from build123d import *

# Parameters (mm, degrees)
CYLINDER002_R             = 3
CYLINDER002_DEPTH         = 10
BOX040_W                  = 56
BOX040_H                  = 10
BOX040_DEPTH              = 122
BOX021_W                  = 47.2
BOX021_H                  = 35
BOX021_DEPTH              = 8
BOX023_W                  = 4.5
BOX023_H                  = 2
BOX023_DEPTH              = 8
BOX022_W                  = 2
BOX022_H                  = 4.5
BOX022_DEPTH              = 8
BOX020_W                  = 17
BOX020_H                  = 5
BOX020_DEPTH              = 12
BOX018_W                  = 48.5
BOX018_H                  = 4.6
BOX018_DEPTH              = 25.5
FUSION005_PLACEMENT_ANGLE = 90
BOX029_W                  = 10
BOX029_H                  = 5
BOX029_DEPTH              = 10
BOX027_W                  = 29.6
BOX027_H                  = 2
BOX027_DEPTH              = 99.5
BOX028_W                  = 10
BOX028_H                  = 5
BOX028_DEPTH              = 10
BOX035_W                  = 10
BOX035_H                  = 77
BOX035_DEPTH              = 10
BOX034_W                  = 10
BOX034_H                  = 74
BOX034_DEPTH              = 10
CUT016_PLACEMENT_ANGLE    = 90
BOX037_W                  = 10
BOX037_H                  = 77
BOX037_DEPTH              = 10
BOX036_W                  = 10
BOX036_H                  = 74
BOX036_DEPTH              = 10
CUT017_PLACEMENT_ANGLE    = 90
BOX039_W                  = 10
BOX039_H                  = 77
BOX039_DEPTH              = 10
BOX038_W                  = 10
BOX038_H                  = 74
BOX038_DEPTH              = 10
CUT018_PLACEMENT_ANGLE    = 180
BOX033_W                  = 10
BOX033_H                  = 77
BOX033_DEPTH              = 10
BOX017_W                  = 10
BOX017_H                  = 74
BOX017_DEPTH              = 10
BOX032_W                  = 39
BOX032_H                  = 10
BOX032_DEPTH              = 10
BOX024_W                  = 50
BOX024_H                  = 39
BOX024_DEPTH              = 8
BOX026_W                  = 72
BOX026_H                  = 18
BOX026_DEPTH              = 1.7
BOX025_W                  = 3
BOX025_H                  = 10
BOX025_DEPTH              = 5.8
ARRAY005_X_COUNT          = 2
ARRAY005_X_PITCH          = 67
CYLINDER001_R             = 1.2
CYLINDER001_DEPTH         = 4
CYLINDER_R                = 2.6
CYLINDER_DEPTH            = 4
ARRAY006_X_COUNT          = 2
ARRAY006_X_PITCH          = 25
ARRAY006_Z_COUNT          = 2
ARRAY006_Z_PITCH          = 95
BOX016_W                  = 114
BOX016_H                  = 50
BOX016_DEPTH              = 144
BOX015_W                  = 120
BOX015_H                  = 42
BOX015_DEPTH              = 150
FILLET001_R               = 7
CHAMFER_SIZE              = 5
FILLET002_R               = 1.5


with BuildPart() as cilindro002:
    # Cylinder002 → Cylinder002 (new body)
    with BuildSketch(Plane(origin=(101.22, 63.68, 142.21), x_dir=(1, 0, 0), z_dir=(0, 0, 1))):
        Circle(CYLINDER002_R)
    extrude(amount=CYLINDER002_DEPTH)


with BuildPart() as cubo021:
    # Box040 → Box040 (new body)
    with BuildSketch(Plane(origin=(11, 81, 19), x_dir=(1, 0, 0), z_dir=(0, 0, 1))):
        with Locations((28, 5)):
            Rectangle(BOX040_W, BOX040_H)
    extrude(amount=BOX040_DEPTH)


with BuildPart() as protoboard:
    # Box021 → Box021 (new body)
    with BuildSketch(Plane.XY):
        with Locations((23.6, 17.5)):
            Rectangle(BOX021_W, BOX021_H)
    extrude(amount=BOX021_DEPTH)


with BuildPart() as obj1:
    # Box023 → Box023 (new body)
    with BuildSketch(Plane(origin=(21.25, 35, 0), x_dir=(1, 0, 0), z_dir=(0, 0, 1))):
        with Locations((2.25, 1)):
            Rectangle(BOX023_W, BOX023_H)
    extrude(amount=BOX023_DEPTH)


with BuildPart() as obj2:
    # Box022 → Box022 (new body)
    with BuildSketch(Plane(origin=(47, 15.25, 0), x_dir=(1, 0, 0), z_dir=(0, 0, 1))):
        with Locations((1, 2.25)):
            Rectangle(BOX022_W, BOX022_H)
    extrude(amount=BOX022_DEPTH)


with BuildPart() as cubo010:
    # Box020 → Box020 (new body)
    with BuildSketch(Plane(origin=(-7, 5, 6.75), x_dir=(1, 0, 0), z_dir=(0, 0, 1))):
        with Locations((8.5, 2.5)):
            Rectangle(BOX020_W, BOX020_H)
    extrude(amount=BOX020_DEPTH)


with BuildPart() as obj3:
    # Box018 → Box018 (new body)
    with BuildSketch(Plane(origin=(0, 0.4, 0), x_dir=(1, 0, 0), z_dir=(0, 0, 1))):
        with Locations((24.25, 2.3)):
            Rectangle(BOX018_W, BOX018_H)
    extrude(amount=BOX018_DEPTH)

    # Fusion005: union Cubo010
    add(cubo010.part)


with BuildPart() as obj3_1:
    # Fusion005 placement: moved
    add(obj3.part.moved(Location((-0.75, 30.25, 7.6))).rotate(Axis((-0.75, 30.25, 7.6), (1, 0, 0)), FUSION005_PLACEMENT_ANGLE))

    # Fusion006: union protoboard, obj1, obj2
    add(protoboard.part)
    add(obj1.part)
    add(obj2.part)


with BuildPart() as obj3_2:
    # Fusion006 placement: moved
    add(obj3_1.part.moved(Location((4, 45, 3))))


with BuildPart() as on_off:
    # Box029 → Box029 (new body)
    with BuildSketch(Plane(origin=(26, -6, 81.5), x_dir=(1, 0, 0), z_dir=(0, 0, 1))):
        with Locations((5, 2.5)):
            Rectangle(BOX029_W, BOX029_H)
    extrude(amount=BOX029_DEPTH)


with BuildPart() as obj4:
    # Box027 → Box027 (new body)
    with BuildSketch(Plane.XY):
        with Locations((14.8, 1)):
            Rectangle(BOX027_W, BOX027_H)
    extrude(amount=BOX027_DEPTH)


with BuildPart() as fusion011:
    # Box028 → Box028 (new body)
    with BuildSketch(Plane(origin=(26, 0.6, 5.5), x_dir=(1, 0, 0), z_dir=(0, 0, 1))):
        with Locations((5, 2.5)):
            Rectangle(BOX028_W, BOX028_H)
    extrude(amount=BOX028_DEPTH)

    # Fusion008: union on_off, obj4
    add(on_off.part)
    add(obj4.part)


with BuildPart() as fusion011_1:
    # Fusion008 placement: moved
    add(fusion011.part.moved(Location((85.8, 76, 4.23))))

    # Fusion011: union obj3
    add(obj3_2.part)


with BuildPart() as cubo016:
    # Box035 → Box035 (new body)
    with BuildSketch(Plane(origin=(0, 10, 140), x_dir=(1, 0, 0), z_dir=(0, 0, 1))):
        with Locations((5, 38.5)):
            Rectangle(BOX035_W, BOX035_H)
    extrude(amount=BOX035_DEPTH)


with BuildPart() as cut016:
    # Box034 → Box034 (new body)
    with BuildSketch(Plane(origin=(-3, 10, 143), x_dir=(1, 0, 0), z_dir=(0, 0, 1))):
        with Locations((5, 37)):
            Rectangle(BOX034_W, BOX034_H)
    extrude(amount=BOX034_DEPTH)

    # Cut016: cut Cubo016
    add(cubo016.part, mode=Mode.SUBTRACT)


with BuildPart() as cut016_1:
    # Cut016 placement: moved
    add(cut016.part.moved(Location((-30, 0, 150))).rotate(Axis((-30, 0, 150), (0, 1, 0)), CUT016_PLACEMENT_ANGLE))


with BuildPart() as cubo018:
    # Box037 → Box037 (new body)
    with BuildSketch(Plane(origin=(0, 10, 140), x_dir=(1, 0, 0), z_dir=(0, 0, 1))):
        with Locations((5, 38.5)):
            Rectangle(BOX037_W, BOX037_H)
    extrude(amount=BOX037_DEPTH)


with BuildPart() as cut017:
    # Box036 → Box036 (new body)
    with BuildSketch(Plane(origin=(-3, 10, 143), x_dir=(1, 0, 0), z_dir=(0, 0, 1))):
        with Locations((5, 37)):
            Rectangle(BOX036_W, BOX036_H)
    extrude(amount=BOX036_DEPTH)

    # Cut017: cut Cubo018
    add(cubo018.part, mode=Mode.SUBTRACT)


with BuildPart() as cut017_1:
    # Cut017 placement: moved
    add(cut017.part.moved(Location((150, 0, 0))).rotate(Axis((150, 0, 0), (0, -1, 0)), CUT017_PLACEMENT_ANGLE))


with BuildPart() as cubo020:
    # Box039 → Box039 (new body)
    with BuildSketch(Plane(origin=(0, 10, 140), x_dir=(1, 0, 0), z_dir=(0, 0, 1))):
        with Locations((5, 38.5)):
            Rectangle(BOX039_W, BOX039_H)
    extrude(amount=BOX039_DEPTH)


with BuildPart() as cut018:
    # Box038 → Box038 (new body)
    with BuildSketch(Plane(origin=(-3, 10, 143), x_dir=(1, 0, 0), z_dir=(0, 0, 1))):
        with Locations((5, 37)):
            Rectangle(BOX038_W, BOX038_H)
    extrude(amount=BOX038_DEPTH)

    # Cut018: cut Cubo020
    add(cubo020.part, mode=Mode.SUBTRACT)


with BuildPart() as cut018_1:
    # Cut018 placement: moved
    add(cut018.part.moved(Location((120, 0, 150))).rotate(Axis((120, 0, 150), (0, 1, 0)), CUT018_PLACEMENT_ANGLE))


with BuildPart() as cubo014:
    # Box033 → Box033 (new body)
    with BuildSketch(Plane(origin=(0, 10, 140), x_dir=(1, 0, 0), z_dir=(0, 0, 1))):
        with Locations((5, 38.5)):
            Rectangle(BOX033_W, BOX033_H)
    extrude(amount=BOX033_DEPTH)


with BuildPart() as obj5:
    # Box017 → Box017 (new body)
    with BuildSketch(Plane(origin=(-3, 10, 143), x_dir=(1, 0, 0), z_dir=(0, 0, 1))):
        with Locations((5, 37)):
            Rectangle(BOX017_W, BOX017_H)
    extrude(amount=BOX017_DEPTH)

    # Cut015: cut Cubo014
    add(cubo014.part, mode=Mode.SUBTRACT)

    # Fusion009: union Cut016, Cut017, Cut018
    add(cut016_1.part)
    add(cut017_1.part)
    add(cut018_1.part)


with BuildPart() as cubo013:
    # Box032 → Box032 (new body)
    with BuildSketch(Plane(origin=(9, 43, 3), x_dir=(1, 0, 0), z_dir=(0, 0, 1))):
        with Locations((19.5, 5)):
            Rectangle(BOX032_W, BOX032_H)
    extrude(amount=BOX032_DEPTH)


with BuildPart() as baseproto:
    # Box024 → Box024 (new body)
    with BuildSketch(Plane(origin=(3, 43, 3), x_dir=(1, 0, 0), z_dir=(0, 0, 1))):
        with Locations((25, 19.5)):
            Rectangle(BOX024_W, BOX024_H)
    extrude(amount=BOX024_DEPTH)

    # Cut014: cut Cubo013
    add(cubo013.part, mode=Mode.SUBTRACT)


with BuildPart() as leds:
    # Box026 → Box026 (new body)
    with BuildSketch(Plane(origin=(-1, 0, 2), x_dir=(1, 0, 0), z_dir=(0, 0, 1))):
        with Locations((36, 9)):
            Rectangle(BOX026_W, BOX026_H)
    extrude(amount=BOX026_DEPTH)


with BuildPart() as soporte_placa_leds:
    # Box025 → Box025 (new body)
    with BuildSketch(Plane(origin=(0, 8, 0), x_dir=(1, 0, 0), z_dir=(0, 0, 1))):
        with Locations((1.5, 5)):
            Rectangle(BOX025_W, BOX025_H)
    extrude(amount=BOX025_DEPTH)

    # Array005 X: soporte_placa_leds ×2


with BuildPart() as soporte_placa_leds_1:
    add(soporte_placa_leds.part)
    with Locations(*[(i * ARRAY005_X_PITCH, 0, 0) for i in range(1, ARRAY005_X_COUNT)]):
        add(soporte_placa_leds.part)

    # Cut012: cut leds
    add(leds.part, mode=Mode.SUBTRACT)


with BuildPart() as soporte_placa_leds_2:
    # Cut012 placement: moved
    add(soporte_placa_leds_1.part.moved(Location((4, 65, 70.25))))


with BuildPart() as cilindro001:
    # Cylinder001 → Cylinder001 (new body)
    with BuildSketch(Plane(origin=(2.6, 0, 2.6), x_dir=(1, 0, 0), z_dir=(0, -1, 0))):
        Circle(CYLINDER001_R)
    extrude(amount=CYLINDER001_DEPTH)


with BuildPart() as array006:
    # Cylinder → Cylinder (new body)
    with BuildSketch(Plane(origin=(2.6, 0, 2.6), x_dir=(1, 0, 0), z_dir=(0, -1, 0))):
        Circle(CYLINDER_R)
    extrude(amount=CYLINDER_DEPTH)

    # Cut013: cut Cilindro001
    add(cilindro001.part, mode=Mode.SUBTRACT)


with BuildPart() as array006_1:
    # Cut013 placement: moved
    add(array006.part.moved(Location((31.199794, 82, -20.171414))))

    # Array006 X: Array006 ×2


with BuildPart() as array006_2:
    add(array006_1.part)
    with Locations(*[(i * ARRAY006_X_PITCH, 0, 0) for i in range(1, ARRAY006_X_COUNT)]):
        add(array006_1.part)

    # Array006 Z: Array006 ×2


with BuildPart() as array006_3:
    add(array006_2.part)
    with Locations(*[(0, 0, i * ARRAY006_Z_PITCH) for i in range(1, ARRAY006_Z_COUNT)]):
        add(array006_2.part)


with BuildPart() as array006_4:
    # Array006 placement: moved
    add(array006_3.part.moved(Location((54.6, 0, 24))))


with BuildPart() as cubo006:
    # Box016 → Box016 (new body)
    with BuildSketch(Plane(origin=(3, 32, 3), x_dir=(1, 0, 0), z_dir=(0, 0, 1))):
        with Locations((57, 25)):
            Rectangle(BOX016_W, BOX016_H)
    extrude(amount=BOX016_DEPTH)


with BuildPart() as closet_bottom_esp8266:
    # Box015 → Box015 (new body)
    with BuildSketch(Plane(origin=(0, 42, 0), x_dir=(1, 0, 0), z_dir=(0, 0, 1))):
        with Locations((60, 21)):
            Rectangle(BOX015_W, BOX015_H)
    extrude(amount=BOX015_DEPTH)

    # Cut010: cut Cubo006
    add(cubo006.part, mode=Mode.SUBTRACT)

    # Fusion010: union obj5, baseProto, soporte_placa_leds, Array006
    add(obj5.part)
    add(baseproto.part)
    add(soporte_placa_leds_2.part)
    add(array006_4.part)

    # Cut019: cut Fusion011
    add(fusion011_1.part, mode=Mode.SUBTRACT)

    # Cut020: cut Cubo021
    add(cubo021.part, mode=Mode.SUBTRACT)

    # Cut021: cut Cilindro002
    add(cilindro002.part, mode=Mode.SUBTRACT)

    # Fillet001
    fillet001_edges = [closet_bottom_esp8266.edges().sort_by_distance(p)[0] for p in [
        (5.5, 82, 70.25),
        (5.5, 82, 76.05),
        (72.5, 82, 70.25),
        (72.5, 82, 76.05),
    ]]
    fillet(fillet001_edges, radius=FILLET001_R)

    # Chamfer
    chamfer_edges = [closet_bottom_esp8266.edges().sort_by_distance(p)[0] for p in [
        (53, 51.625, 3),
        (53, 73.375, 3),
    ]]
    chamfer(chamfer_edges, length=CHAMFER_SIZE)

    # Fillet002
    fillet002_edges = [closet_bottom_esp8266.edges().sort_by_distance(p)[0] for p in [
        (120, 79.1, 19.73),
        (120, 76.6, 14.73),
        (120, 79.1, 9.73),
        (120, 81.6, 14.73),
        (120, 72.5, 85.73),
        (120, 75, 90.73),
        (120, 72.5, 95.73),
        (120, 70, 90.73),
        (0, 68.5, 18.1),
        (0, 62.5, 20.6),
        (0, 56.5, 18.1),
        (0, 62.5, 15.6),
    ]]
    fillet(fillet002_edges, radius=FILLET002_R)


solid = closet_bottom_esp8266.part
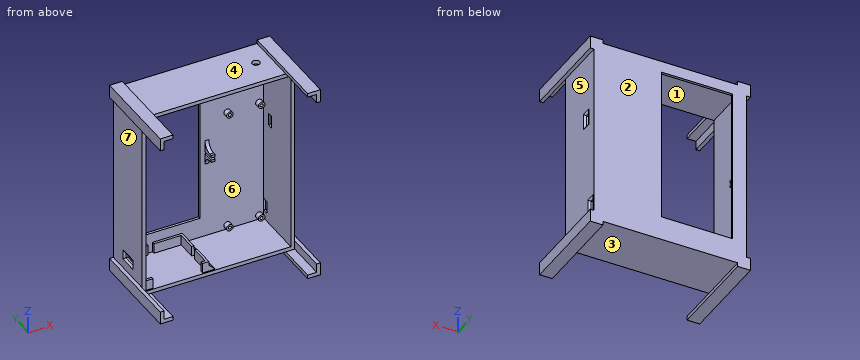
CAD build for the part. Positions are in the model's coordinates, mm. Face numbers are marked on the shaded views. A direction names the side the tool comes from. Give positions to 0.01 mm unless a question says otherwise; leave off trailing zeros. Order: outer loops, then holes, each group sorted by start corner. A loop starts at its lowest first (then second) coordinate and runs counter-clockwise, first axis right, second up. Notation, with made-up numbers: (-17, 15) - (4, 15) arc R31 cw to (4, 45) - close; hole circle Ø4 at (-2.5, -28). An arc over 180 degrees is marked (long way). Write each question's results on one line, items separated by ' | '.
1. 3-axis set-ups, long thin cutter, end or side, ignore diameter. For the marked faces 5, 6 and 7: which of +Z, -Z, +X, -X, +Y, -Y reach the whole face in a straight line?
Calculated:
face 5: +X, +Y, -Y | face 6: -Y | face 7: -X, +Y, -Y
2. Pull direction Z, two halves, no side cores. Call the marked faces 1, 2, 3 and 4: released by +Z, released by -Z, zero draft, split by the parting line, or undercut.
Calculated:
face 1: undercut | face 2: zero draft | face 3: released by -Z | face 4: released by +Z
3. Probe L1, parallel to Z at x = 43, y = 56; L2, parallel to X at y = 14, z = 145.5; L3, parallel to X at y = 65.5, z = 46.5. List the from-to ranges inside material, lowest first. Write a range as from..to.
Calculated:
L1: z = 0..3, 147..150 | L2: x = -3..0, 120..123 | L3: x = 0..3, 117..120
4. Saw through at C-C on z = 131. List the corners of the cut face in (x, y).
Calculated:
outline: (0, 42) - (3, 42) - (3, 82) - (11, 82) - (11, 84) - (0, 84) - close; (67, 82) - (117, 82) - (117, 42) - (120, 42) - (120, 84) - (67, 84) - close
5. Saw through at D-D on y = 17. List the corners of the cut face in (x, z), and give its area (3 significant figures).
Calculated:
outline: (-3, -3) - (7, -3) - (7, 0) - (0, 0) - (0, 7) - (-3, 7) - close; (-3, 143) - (0, 143) - (0, 150) - (7, 150) - (7, 153) - (-3, 153) - close; (113, -3) - (123, -3) - (123, 7) - (120, 7) - (120, 0) - (113, 0) - close; (113, 150) - (120, 150) - (120, 143) - (123, 143) - (123, 153) - (113, 153) - close | area: 204 mm2
6. Pin check, flat tips, straight feed: pin 1 (1 mm diameter, centred on y = 43.5, z = 9, fed in from -X); pin 2 (3 mm diameter, centred on x = 87, z = 99.5, fed in from -Y); pin 3 (0.6 mm diameter, centred on y = 81, z = 8, fed in from +X). Stop position of each tip, or through.
Calculated:
pin 1: stops at x = 0 | pin 2: stops at y = 78 | pin 3: stops at x = 120
7. Saw through at A-A on x = 101.22. List the corners of the cut face in (y, z), and give its area (3 significant figures).
Calculated:
outline: (42, 0) - (84, 0) - (84, 150) - (66.68, 150) - (66.68, 147) - (82, 147) - (82, 3) - (42, 3) - close; (42, 147) - (60.68, 147) - (60.68, 150) - (42, 150) - close | area: 522 mm2
